```python
from build123d import *

# Parameters (mm, degrees)
BOSS_EXTRUDE1_DEPTH = 10
SKETCH2_R           = 10
CUT_EXTRUDE2_DEPTH  = 5
FILLET1_R           = 2


with BuildPart() as part:
    # Sketch1 → Boss-Extrude1 (new body)
    with BuildSketch(Plane.XY):
        with BuildLine():
            Line((-90, -100), (90, -100))
            ThreePointArc((90, -100), (97.071067812, -97.071067812), (100, -90))
            Line((100, -90), (100, 90))
            ThreePointArc((100, 90), (97.071067812, 97.071067812), (90, 100))
            Line((90, 100), (-90, 100))
            ThreePointArc((-90, 100), (-97.071067812, 97.071067812), (-100, 90))
            Line((-100, 90), (-100, -90))
            ThreePointArc((-100, -90), (-97.071067812, -97.071067812), (-90, -100))
        make_face()
    extrude(amount=BOSS_EXTRUDE1_DEPTH)

    # Sketch2 → Cut-Extrude2 (cut)
    with BuildSketch(Plane.XY.offset(10)):
        Circle(SKETCH2_R)
    extrude(amount=-CUT_EXTRUDE2_DEPTH, mode=Mode.SUBTRACT)

    # Fillet1
    fillet1_edges = [part.edges().sort_by_distance(p)[0] for p in [
        (-10, 0, 5),
    ]]
    fillet(fillet1_edges, radius=FILLET1_R)


solid = part.part
```
Check sheet for the modelled part. Datum: model origin and axes. Units: mm. A direction names the side the tool comes from. Coordinates: 2 decimals unless noted, no trailing zeros. Order: outer loops, then holes, each group sorted by start corner. A loop starts at its lowest first (then second) coordinate and runs counter-clockwise, first axis right, second up. Notation, with made-up numbers: (8, -28) -> (62, -28) arc R16 cw to (62, -19) -> close; hole circle Ø1 at (76.25, -16.75). An arc over 180 degrees is marked (long way). Write item = value, one per line. Start each with the question number.
1) Mould release check, pull along Y, two halves, no side actions. Record for faces 1 (the cylindrical face through (97.15, 96.99, 4.93)), 2 (the flat face through (-1, 1, 0)), 3 (the flat face through (0, 0, 5)): +Y half, -Y half, draft (parallel to the pull), parting line (faces both ways), or undercut.
2) Go/stop test with flat-tipped pins: P1, Ø5, axis at x = 13.5, y = -49, coming from the -Z side; P2, Ø8, axis at x = -1.5, y = 3, coming from the +Z side; P3, Ø18, axis at x = 0, y = 0, coming from the +Z side. Record where each tip stops, or that it passes through.
3) Material ranges on L1, parallel to Y at x = 0, z = 8.5, recorded low to high.
4) Access from +Z, -Z, +X, -X, +Y, -Y to the whole of each face (thin tool, end or side, straight path). Record for faces 4 (the cylindrical face through (96.99, -97.15, 4.93)), 5 (the cylindrical face through (-2.17, -9.76, 8.52)).
5) Cross-section at A-A (y = 0). Enter the section's corners in (x, z), then the cut area to 3 significant figures.
Ans:
q1.face_1 = +Y half
q1.face_2 = draft
q1.face_3 = undercut
q2.P1 = 0
q2.P2 = 5
q2.P3 = 5.27
q3.L1 = -100 to -10, 10 to 100
q4.face_4 = +Z, -Z, +X, -Y
q4.face_5 = +Z
q5.outline = (-100, 0) -> (100, 0) -> (100, 10) -> (10, 10) -> (10, 7) arc R2 cw to (8, 5) -> (-8, 5) arc R2 cw to (-10, 7) -> (-10, 10) -> (-100, 10) -> close
q5.area = 1,900 mm²
